The drawing under review shows one solid part. Ordinate dimensions are in mm from its lowest x, y, z. A direction names the side the tool comes from. Coordinates: 2 decimals unless noted, no trailing zeros. Order: outer loops, then holes, each group sorted by start corner. A loop starts at its lowest first (then second) coordinate and runs counter-clockwise, first axis right, second up. Notation, with made-up numbers: (63.5, -32.75) -> (84.5, -32.75) arc R22 ccw to (84.5, -15.75) -> close; hole circle Ø2 at (2, 5.25). An arc over 180 degrees is marked (long way). Write item = value, one per line.
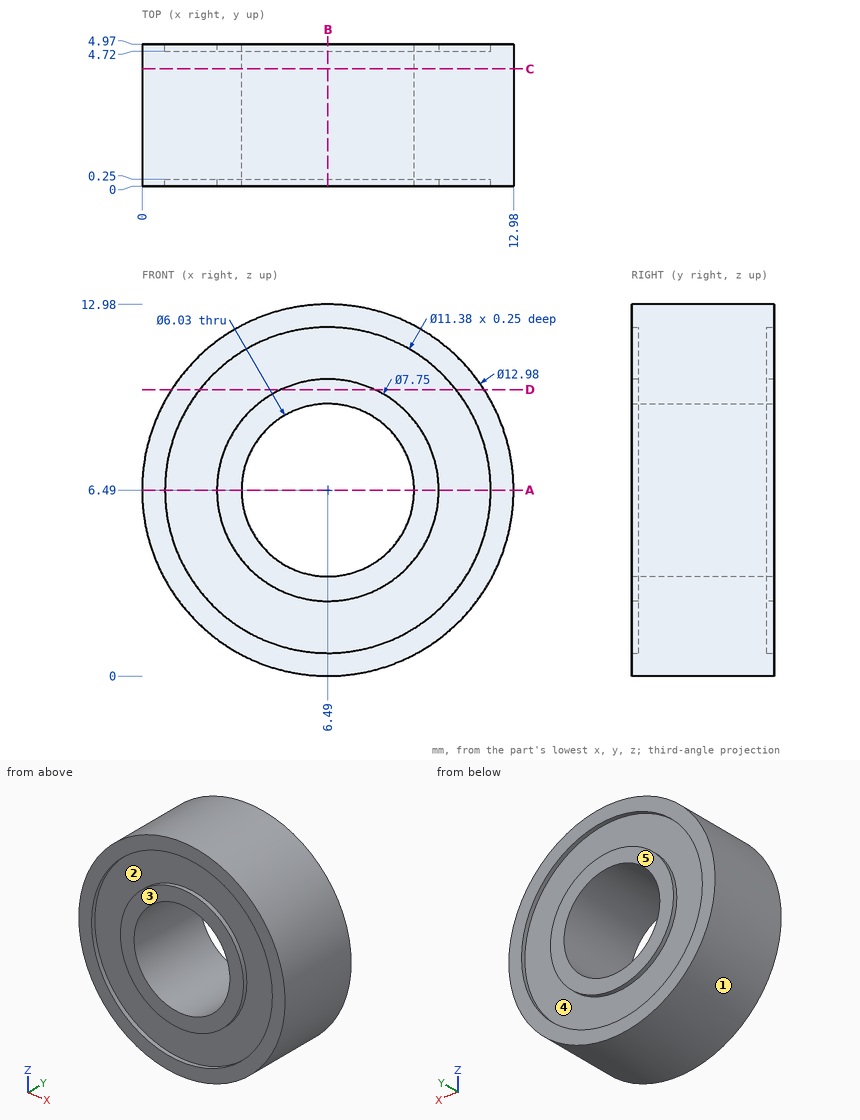
(1) The part is to be moulded in two halves that separate along Z. For the marked faces 1, 2 and 3, say which applies: released by +Z, released by -Z, zero draft, split by the parting line, or undercut.
Report:
face_1 = split by the parting line
face_2 = undercut
face_3 = zero draft
(2) We need section B-B (x = 6.49). Write out the cut boundary in (y, z) (3 decimals).
Report:
outline = (0, 0) -> (4.97, 0) -> (4.97, 0.8) -> (4.72, 0.8) -> (4.72, 2.615) -> (4.97, 2.615) -> (4.97, 3.475) -> (0, 3.475) -> (0, 2.615) -> (0.25, 2.615) -> (0.25, 0.8) -> (0, 0.8) -> close; (0, 9.505) -> (4.97, 9.505) -> (4.97, 10.365) -> (4.72, 10.365) -> (4.72, 12.18) -> (4.97, 12.18) -> (4.97, 12.98) -> (0, 12.98) -> (0, 12.18) -> (0.25, 12.18) -> (0.25, 10.365) -> (0, 10.365) -> close
(3) We need section C-C (y = 4.1). Write out the cut boundary in (x, z) (3 decimals).
Report:
outline = circle Ø12.98 at (6.49, 6.49); hole circle Ø6.03 at (6.49, 6.49)
(4) For the marked faces 4 and 5, list the 3-axis set-ups (+Z, -Z, +X, -X, +Y, -Y) from which the entire face can be reached by the end or side of a thin tool; tool diameter is ignored.
Report:
face_4 = +Y
face_5 = +Z, -Z, +X, -X, +Y
(5) We need section A-A (z = 6.49). Write out the cut boundary in (x, y) (3 decimals), and give its area (3 significant figures).
Report:
outline = (0, 0) -> (0.8, 0) -> (0.8, 0.25) -> (2.615, 0.25) -> (2.615, 0) -> (3.475, 0) -> (3.475, 4.97) -> (2.615, 4.97) -> (2.615, 4.72) -> (0.8, 4.72) -> (0.8, 4.97) -> (0, 4.97) -> close; (9.505, 0) -> (10.365, 0) -> (10.365, 0.25) -> (12.18, 0.25) -> (12.18, 0) -> (12.98, 0) -> (12.98, 4.97) -> (12.18, 4.97) -> (12.18, 4.72) -> (10.365, 4.72) -> (10.365, 4.97) -> (9.505, 4.97) -> close
area = 32.7 mm²
(6) Insertion check: pin 1 (5.5 mm diameter, centred on x = 6.5, z = 9, fed in from +Y). The pin has a flat end and moves straight along its axis. Give the tip position at first contact, or say it passes through.
Report:
pin_1 = 4.97
(7) For L1, parallel to Z at x = 6.49, y = 0.1 (3 decimals); L2, parallel to Z at x = 7.5, y = 4.75, list the stretches that pass through material, from the lowest coordinate up.
Report:
L1 = 0 to 0.8, 2.615 to 3.475, 9.505 to 10.365, 12.18 to 12.98
L2 = 0.08 to 0.89, 2.75 to 3.65, 9.33 to 10.23, 12.09 to 12.9
(8) We need section D-D (z = 10). Write out the cut boundary in (x, y).
Report:
outline = (1.03, 0) -> (2.01, 0) -> (2.01, 0.25) -> (4.85, 0.25) -> (4.85, 0) -> (8.13, 0) -> (8.13, 0.25) -> (10.97, 0.25) -> (10.97, 0) -> (11.95, 0) -> (11.95, 4.97) -> (10.97, 4.97) -> (10.97, 4.72) -> (8.13, 4.72) -> (8.13, 4.97) -> (4.85, 4.97) -> (4.85, 4.72) -> (2.01, 4.72) -> (2.01, 4.97) -> (1.03, 4.97) -> close
